from build123d import *

# Parameters (mm, degrees)
F0_R     = 7.9375
F1_DEPTH = 22
F2_R     = 6
F3_DEPTH = 78
F4_R     = 6
F4_R_2   = 4.5
F5_DEPTH = 25
F6_SIZE2 = 5.4949548389
F6_SIZE  = 2


# Not quite as in the source:
# - a feature names something its author has since deleted; it is built from what else it names


with BuildPart() as f1:
    # F0 (on Front) → F1 (new body)
    with BuildSketch(Plane.XZ):
        Circle(F0_R)
    extrude(amount=F1_DEPTH)

    # F2 (on Front) → F3 (join)
    with BuildSketch(Plane.XZ):
        Circle(F2_R)
    extrude(amount=-F3_DEPTH)

    # F4 (on face) → F5 (cut)
    with BuildSketch(Plane(origin=(0, 78, 0), x_dir=(-1, 0, 0), z_dir=(0, 1, 0))):
        Circle(F4_R)
        Circle(F4_R_2, mode=Mode.SUBTRACT)
    extrude(amount=-F5_DEPTH, mode=Mode.SUBTRACT)

    # F6
    f6_edges = [f1.edges().sort_by_distance(p)[0] for p in [
        (-7.9375, -22, 0),
    ]]
    f6_side = f1.faces().sort_by_distance((0, -22, 0))[0]
    chamfer(f6_edges, length=F6_SIZE, length2=F6_SIZE2, reference=f6_side)


solid = f1.part
Work out the finished part from the listing and answer in its coordinate system (mm). A direction names the side the tool comes from. Coordinates: 2 decimals unless noted, no trailing zeros. Write each loop counter-clockwise with the first axis right and the second up, starting at its lowest first coordinate (ties: lowest second). Pieces come first, ordered by that corner, then holes. Notation, with made-up numbers: M 10,-31.5 L 64,-31.5 A27 cw 64,-6.5 Z; hole C 5,-12 d6. An arc over 180 degrees is marked long. Use one line per item in the form item = value. Start each with the question number.
1. A tool of negligible diameter and unlimited length cuts with its end or side. For faces 1 (the face through (-1.72, -8.14, -7.75)), 2 (the face through (-2, 0, 6)), from which of +Z, -Z, +X, -X, +Y, -Y can it reach the whole face along a straight path? Write none if from no direction.
2. The part is cut by section C-C (y = 21). Give the vertices of the cut face in (x, z).
3. The part is cut by section D-D (y = -14). Give the vertices of the cut face in (x, z) (1 decimal), plus the area to 3 significant figures.
4. The part is cut by section B-B (x = 0). Give the vertices of the cut face in (y, z), plus the area to 3 significant figures.
5. The part is cut by section A-A (z = 0). Give the vertices of the cut face in (x, y), plus the area to 3 significant figures.
6. Straight lines are drawn through the part: probe 1 along Y at (x, z) = (5, -2.75); probe 2 along Z at (x, y) = (0, 30); probe 3 along X at (y, z) = (-12, 0.25). For each, find the intervals that lie inside material, in ascending order. Write a range as from..to.
7. Each of these flat-tipped pins is pushed along its axis until it touches: P1, Ø6, axis at y = 26, z = 6, coming from the -X side; P2, Ø5, axis at y = 51, z = -4.5, coming from the -X side; P3, Ø1, axis at x = -4, y = 12.5, coming from the -Z side. Where does it stop, or does it pass through?
Evaluation:
q1.face_1 = +Y, -Y
q1.face_2 = +Y
q2.outline = C 0,0 d12
q3.outline = C 0,0 d15.9
q3.area = 198 mm^2
q4.outline = M -22,-5.94 L -16.51,-7.94 L 0,-7.94 L 0,-6 L 53,-6 L 53,-4.5 L 78,-4.5 L 78,4.5 L 53,4.5 L 53,6 L 0,6 L 0,7.94 L -16.51,7.94 L -22,5.94 Z
q4.area = 1,200 mm^2
q5.outline = M -7.94,-16.51 L -5.94,-22 L 5.94,-22 L 7.94,-16.51 L 7.94,0 L 6,0 L 6,53 L 4.5,53 L 4.5,78 L -4.5,78 L -4.5,53 L -6,53 L -6,0 L -7.94,0 Z
q5.area = 1,200 mm^2
q6.probe_1 = -22..53
q6.probe_2 = -6..6
q6.probe_3 = -7.93..7.93
q7.P1 = -5.2
q7.P2 = -5.66
q7.P3 = -4.87
